from build123d import *

# Parameters (mm, degrees)
SKICA1_R                = 60
SKICA1_R_2              = 15
P_IDAT_VYSUNUT_M1_DEPTH = 2
SKICA2_R                = 60
SKICA2_R_2              = 58
P_IDAT_VYSUNUT_M2_DEPTH = 10
ZKOSEN_1_SIZE           = 1
ZKOSEN_2_SIZE           = 1
ZKOSEN_3_SIZE           = 1


with BuildPart() as part:
    # Skica1 → Přidat vysunutím1 (new body)
    with BuildSketch(Plane(origin=(0, 0, 0), x_dir=(1, 0, 0), z_dir=(0, 1, 0))):
        with Locations(Location((0, 0, 0), (0, 0, 270))):
            Circle(SKICA1_R)
        with Locations(Location((0, 0, 0), (0, 0, 270))):
            Circle(SKICA1_R_2, mode=Mode.SUBTRACT)
    extrude(amount=P_IDAT_VYSUNUT_M1_DEPTH)

    # Skica2 → Přidat vysunutím2 (add)
    with BuildSketch(Plane(origin=(0, 2, 0), x_dir=(1, 0, 0), z_dir=(0, 1, 0))):
        with Locations(Location((0, 0, 0), (0, 0, 270))):
            Circle(SKICA2_R)
        with Locations(Location((0, 0, 0), (0, 0, 270))):
            Circle(SKICA2_R_2, mode=Mode.SUBTRACT)
    extrude(amount=P_IDAT_VYSUNUT_M2_DEPTH)

    # Zkosení1
    zkosen_1_edges = [part.edges().sort_by_distance(p)[0] for p in [
        (0, 2, -58),
    ]]
    chamfer(zkosen_1_edges, length=ZKOSEN_1_SIZE)

    # Zkosení2
    zkosen_2_edges = [part.edges().sort_by_distance(p)[0] for p in [
        (0, 0, -60),
    ]]
    chamfer(zkosen_2_edges, length=ZKOSEN_2_SIZE)

    # Zkosení3
    zkosen_3_edges = [part.edges().sort_by_distance(p)[0] for p in [
        (0, 12, -60),
    ]]
    chamfer(zkosen_3_edges, length=ZKOSEN_3_SIZE)


solid = part.part
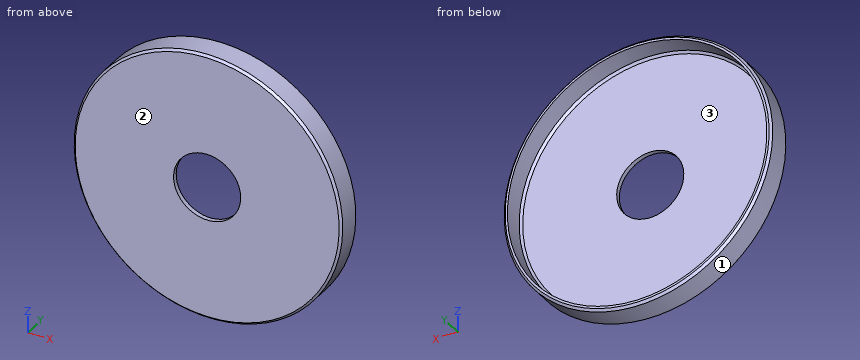
Read the model definition and answer for the solid it produces. Units are mm, in the model's axes. Face numbers are marked on the shaded views. Give positions to 0.01 mm unless a question says otherwise; leave off trailing zeros. Write each loop counter-clockwise with the first axis right and the second up, starting at its lowest first coordinate (ties: lowest second). Pieces come first, ordered by that corner, then holes. Notation, with made-up numbers: (43.25, -4) - (49.25, -4) arc R34 cw to (49.25, 27) - close; hole circle Ø1 at (71, 2.5). An arc over 180 degrees is marked (long way). Answer in a Markdown table with one row per item. Add a question column.
Item 1: Section C-C, the plane y = 5.25 is taken. Write down the section's boundary in (x, z), and give its area (3 significant figures).
Item 2: Section B-B, the plane x = 0 is taken. Write down the section's boundary in (y, z), and give its area (3 significant figures).
Item 3: Section A-A, the plane z = 0 is taken. Write down the section's boundary in (x, y), and give its area (3 significant figures).
Item 4: Find the intervals of material crossed by L1, parallel to X at y = 1.4, z = 0; L2, parallel to Y at x = -12, z = 51; L3, parallel to Z at x = -39.5, y = 2.5, in increasing order.
Item 5: Determine the mould class of the marked faces 1, 2 and 3 for opening direction Z: pulls with the +Z half, pulls with the -Z half, needs draft (parallel to the pull), parting line crosses it, or undercut.
Item 6: Flat-ended cylindrical pins translate along their axes: P1, Ø5, axis at y = 2, z = 18.5, coming from the +X side; P2, Ø12, axis at x = 4, z = 13.5, coming from the -Y side; P3, Ø2, axis at y = 7, z = -14, coming from the -X side; P4, Ø24, axis at x = 0, z = 0, coming from the -Y side. Find the tip coordinate at first contact, or state that the pin passes through.
Recorded:
| question | item | result |
|---|---|---|
| 1 | outline | circle Ø120 at (0, 0); hole circle Ø116 at (0, 0) |
| 1 | area | 741 mm2 |
| 2 | outline | (0, -59) - (1, -60) - (11, -60) - (12, -59) - (12, -58) - (3, -58) - (2, -57) - (2, -15) - (0, -15) - close; (0, 15) - (2, 15) - (2, 57) - (3, 58) - (12, 58) - (12, 59) - (11, 60) - (1, 60) - (0, 59) - close |
| 2 | area | 219 mm2 |
| 3 | outline | (-60, 1) - (-59, 0) - (-15, 0) - (-15, 2) - (-57, 2) - (-58, 3) - (-58, 12) - (-59, 12) - (-60, 11) - close; (15, 0) - (59, 0) - (60, 1) - (60, 11) - (59, 12) - (58, 12) - (58, 3) - (57, 2) - (15, 2) - close |
| 3 | area | 219 mm2 |
| 4 | L1 | x = -60 to -15, 15 to 60 |
| 4 | L2 | y = 0 to 2 |
| 4 | L3 | z = -45.16 to -41.79, 41.79 to 45.16 |
| 5 | face 1 | parting line crosses it |
| 5 | face 2 | needs draft |
| 5 | face 3 | undercut |
| 6 | P1 | stops at x = 57.83 |
| 6 | P2 | stops at y = 0 |
| 6 | P3 | stops at x = -58.57 |
| 6 | P4 | passes through |
